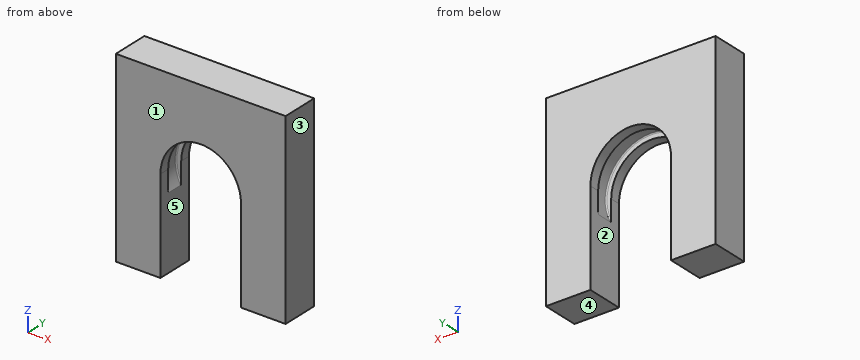
```python
from build123d import *

# Parameters (mm, degrees)
F1_DEPTH = 17.5
F4_R     = 1
F5_R     = 1


with BuildPart() as f1:
    # F0 (on Front) → F1 (new body, symmetric)
    with BuildSketch(Plane.XZ):
        with BuildLine():
            ThreePointArc((-38, 0), (0, 38), (38, 0))
            Line((38, 0), (38, -88.42741))
            Line((38, -88.42741), (80, -88.42741))
            Line((80, -88.42741), (80, 88.42741))
            Line((80, 88.42741), (-80, 88.42741))
            Line((-80, 88.42741), (-80, -88.42741))
            Line((-80, -88.42741), (-38, -88.42741))
            Line((-38, -88.42741), (-38, 0))
        make_face()
    extrude(amount=F1_DEPTH, both=True)

    # F2 (on Right) → F3 (revolve, cut)
    with BuildSketch(Plane.YZ):
        Polygon((-8, 43), (-8, 32.880556), (8, 32.880556), (8, 43), (0, 43), align=None)
    revolve(axis=Axis((0, 0, 0), (0, -1, 0)), mode=Mode.SUBTRACT)

    # F4
    f4_edges = [f1.edges().sort_by_distance(p)[0] for p in [
        (0, 8, 43),
    ]]
    fillet(f4_edges, radius=F4_R)

    # F5
    f5_edges = [f1.edges().sort_by_distance(p)[0] for p in [
        (0, -8, 43),
    ]]
    fillet(f5_edges, radius=F5_R)


solid = f1.part
```
Here's how the part is built. I have some questions about the finished solid (model axes, mm). Face numbers are marked on the shaded views. A direction names the side the tool comes from. Give positions to 0.01 mm unless a question says otherwise; leave off trailing zeros. Order: outer loops, then holes, each group sorted by start corner. A loop starts at its lowest first (then second) coordinate and runs counter-clockwise, first axis right, second up. Notation, with made-up numbers: M 43,14.25 L 70,14.25 A18 cw 70,29.25 Z; hole C 65,59 d8. An arc over 180 degrees is marked long. Use a Markdown table: item, result. Add a question column.
1. I need wall thicknesses on probe 1 along X at (y, z) = (3, 0); probe 2 along X at (y, z) = (13, -54); probe 3 along Z at (x, y) = (0, -3). Which ranges of each line are inside material? Lowest first, please. Write a range as from..to.
2. Suppose I cut it at A-A (z = -46). List the corners of the cut face in (x, y) for me, and give its area (3 significant figures).
3. For pin 1 Ø5 at (x, y) = (-26.5, 9.5) entering from -Z, with a flat end and sliding along its axis, tell me the tip position at first contact or that it passes through.
4. Suppose I cut it at B-B (x = 0). List the corners of the cut face in (y, z) for me, and give its area (3 significant figures).
5. If we mould it in two halves opening along X, with no side actions, what happens to the marked faces 1, 2 and 3? For each: +X half, -X half, draft (parallel to the pull), parting line (faces both ways), or undercut.
6. On a 3-axis mill with a long thin cutter (end or side, diameter ignored), from which of +Z, -Z, +X, -X, +Y, -Y can I reach the whole of each face in a straight line? I mean the marked faces 4 and 5. Say none if no direction works.
7. Suppose I cut it at C-C (y = -5). List the corners of the cut face in (x, z) for me.
Results list:
| question | item | result |
|---|---|---|
| 1 | probe 1 | x = -80..-43, 43..80 |
| 1 | probe 2 | x = -80..-38, 38..80 |
| 1 | probe 3 | z = 43..88.43 |
| 2 | outline | M -80,-17.5 L -38,-17.5 L -38,17.5 L -80,17.5 Z; M 38,-17.5 L 80,-17.5 L 80,17.5 L 38,17.5 Z |
| 2 | area | 2,940 mm² |
| 3 | pin 1 | stops at z = 24.56 |
| 4 | outline | M -17.5,38 L -8,38 L -8,42 A1 cw -7,43 L 7,43 A1 cw 8,42 L 8,38 L 17.5,38 L 17.5,88.43 L -17.5,88.43 Z |
| 4 | area | 1,690 mm² |
| 5 | face 1 | draft |
| 5 | face 2 | undercut |
| 5 | face 3 | +X half |
| 6 | face 4 | -Z, +X, -X, +Y, -Y |
| 6 | face 5 | -Z, +Y, -Y |
| 7 | outline | M -80,-88.43 L -38,-88.43 L -38,-20.12 A43 cw long 38,-20.12 L 38,-88.43 L 80,-88.43 L 80,88.43 L -80,88.43 Z |
